Can you work these out from the model? Positions are in its coordinate system, mm. A direction names the side the tool comes from. Coordinates: 2 decimals unless noted, no trailing zeros. Order: outer loops, then holes, each group sorted by start corner. A loop starts at its lowest first (then second) coordinate and runs counter-clockwise, first axis right, second up. Notation, with made-up numbers: (55, 11) -> (85, 11) arc R27 cw to (85, 32) -> close; hole circle Ø5 at (11.5, -6). An arc over 180 degrees is marked (long way). Answer in a Markdown table with one row per item.
```python
from build123d import *

# Parameters (mm, degrees)
SALIENTE_EXTRUIR1_DEPTH = 10
CROQUIS2_R              = 2.5
CORTAR_EXTRUIR1_DEPTH   = 1
CROQUIS3_R              = 2.5
CORTAR_EXTRUIR2_DEPTH   = 1


with BuildPart() as part:
    # Croquis1 → Saliente-Extruir1 (new body)
    with BuildSketch(Plane(origin=(0, 0, 0), x_dir=(1, 0, 0), z_dir=(0, 1, 0))):
        with BuildLine():
            ThreePointArc((-25.446754953, 16.759256359), (-25.153861734, 17.46636314), (-24.446754953, 17.759256359))
            Line((-24.446754953, 17.759256359), (14.553245047, 17.759256359))
            Line((14.553245047, 17.759256359), (14.553245047, 16.759256359))
            Line((14.553245047, 16.759256359), (-24.446754953, 16.759256359))
            Line((-24.446754953, 16.759256359), (-24.446754953, -22.240743641))
            Line((-24.446754953, -22.240743641), (-25.446754953, -22.240743641))
            Line((-25.446754953, -22.240743641), (-25.446754953, 16.759256359))
        make_face()
    extrude(amount=SALIENTE_EXTRUIR1_DEPTH)

    # Croquis2 → Cortar-Extruir1 (cut)
    with BuildSketch(Plane.XY.offset(-16.759256359)):
        with Locations((4.553245047, 5)):
            Circle(CROQUIS2_R)
        with Locations((-15.446754953, 5)):
            Circle(CROQUIS2_R)
    extrude(amount=-CORTAR_EXTRUIR1_DEPTH, mode=Mode.SUBTRACT)

    # Croquis3 → Cortar-Extruir2 (cut)
    with BuildSketch(Plane(origin=(-24.446754953, 0, 0), x_dir=(0, 0, -1), z_dir=(1, 0, 0))):
        with Locations((-12.240743641, 5)):
            Circle(CROQUIS3_R)
        with Locations((7.759256359, 5)):
            Circle(CROQUIS3_R)
    extrude(amount=-CORTAR_EXTRUIR2_DEPTH, mode=Mode.SUBTRACT)


solid = part.part
```
(1) Will these pins go through, and if not, where does the flat tip stop? pin 1 Ø5 at (y, z) = (3.5, 2.5) entering from +X; pin 2 Ø6 at (x, y) = (-3, 8.5) entering from +Z.
Response values:
| item | result |
|---|---|
| pin 1 | x = -24.45 |
| pin 2 | z = -16.76 |
(2) Suppose I cut it at B-B (z = -6.5). Please give me the cut outline in (x, y).
Response values:
| item | result |
|---|---|
| outline | (-25.45, 0) -> (-24.45, 0) -> (-24.45, 2.84) -> (-25.45, 2.84) -> close; (-25.45, 7.16) -> (-24.45, 7.16) -> (-24.45, 10) -> (-25.45, 10) -> close |
(3) Suppose I cut it at C-C (y = 8.5). Please give me the cut outline in (x, z).
Response values:
| item | result |
|---|---|
| outline | (-25.45, -16.76) arc R1 ccw to (-24.45, -17.76) -> (14.55, -17.76) -> (14.55, -16.76) -> (-24.45, -16.76) -> (-24.45, 22.24) -> (-25.45, 22.24) -> close |
(4) Suppose I cut it at D-D (z = 18). Please give me the cut outline in (x, y).
Response values:
| item | result |
|---|---|
| outline | (-25.45, 0) -> (-24.45, 0) -> (-24.45, 10) -> (-25.45, 10) -> close |
(5) On a 3-axis mill with a long thin cutter (end or side, diameter ignored), from which of +Z, -Z, +X, -X, +Y, -Y can I reach the whole of each face in a straight line? I mean faces 4 (the flat face through (-25.447, 5, 3)), 5 (the flat face through (-24.447, 5, 2)). Say none if no direction works.
Response values:
| item | result |
|---|---|
| face 4 | +Z, -Z, -X, +Y, -Y |
| face 5 | +Z, +X, +Y, -Y |
(6) We'd pull the mould along Y, two halves only. Please class faces 1 (the cylindrical face through (-25.16, 4.93, -17.46)), 2 (the cylindrical face through (-17.29, 6.69, -17.25)), 3 (the flat face through (-25, 10, -7)): +Y half, -Y half, draft (parallel to the pull), parting line (faces both ways), or undercut.
Response values:
| item | result |
|---|---|
| face 1 | draft |
| face 2 | undercut |
| face 3 | +Y half |
(7) Suppose I cut it at A-A (y = 5). Please give me the cut outline in (x, z), and give its area (3 significant figures).
Response values:
| item | result |
|---|---|
| outline | (-25.45, -16.76) arc R1 ccw to (-24.45, -17.76) -> (-17.95, -17.76) -> (-17.95, -16.76) -> (-24.45, -16.76) -> (-24.45, -10.26) -> (-25.45, -10.26) -> close; (-25.45, -5.26) -> (-24.45, -5.26) -> (-24.45, 9.74) -> (-25.45, 9.74) -> close; (-25.45, 14.74) -> (-24.45, 14.74) -> (-24.45, 22.24) -> (-25.45, 22.24) -> close; (-12.95, -17.76) -> (2.05, -17.76) -> (2.05, -16.76) -> (-12.95, -16.76) -> close; (7.05, -17.76) -> (14.55, -17.76) -> (14.55, -16.76) -> (7.05, -16.76) -> close |
| area | 58.8 mm2 |
(8) I need wall thicknesses on line 1 (Z direction, x = -23, y = 5.25); line 2 (X direction, y = 2.5, z = -12.5). Which ranges of each line are inside material? Lowest first, please. Write a range as [from, to].
Response values:
| item | result |
|---|---|
| line 1 | [-17.76, -16.76] |
| line 2 | [-25.45, -24.45] |
